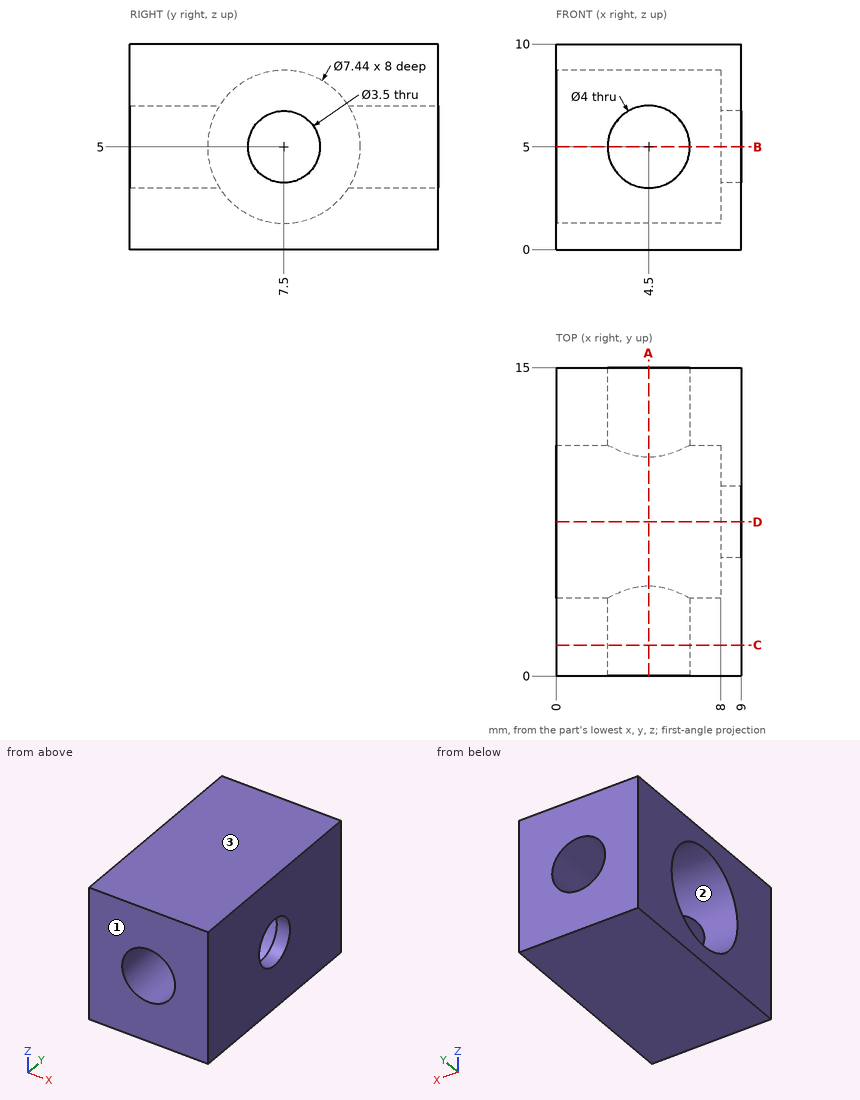
Print and shaded views of the part. All mm, measured from the part's lowest x, y and z. Coordinates: 2 decimals unless noted, no trailing zeros. Order: outer loops, then holes, each group sorted by start corner. A loop starts at its lowest first (then second) coordinate and runs counter-clockwise, first axis right, second up. Notation, with made-up numbers: (-21.5, 24.5) - (15.5, 24.5) arc R16 ccw to (15.5, 32.5) - close; hole circle Ø6 at (68.25, 5). An arc over 180 degrees is marked (long way). Return JSON: item names as keys, results as strings. Group by question number.
Item 1: Cut at C-C (y = 1.5). List the corners of the cut face in (x, z), plus the area to 3 significant figures.
Item 2: Cut at B-B (z = 5). List the corners of the cut face in (x, y), plus the area to 3 significant figures.
Item 3: Pull direction Y, two halves, no side cores. Call the marked faces 1, 2 and 3: pulls with the +Y half, pulls with the -Y half, needs draft (parallel to the pull), parting line crosses it, or undercut.
Item 4: Cut at A-A (x = 4.5). List the corners of the cut face in (y, z).
Item 5: Cut at D-D (y = 7.5). List the corners of the cut face in (x, z).
Item 6: Drill centre lines: probe 1 along X at (y, z) = (2.05, 5); probe 2 along Z at (x, y) = (4.5, 2.7); probe 3 along Z at (x, y) = (4.25, 7.5). Where is each one in solid material? Low to high. Write a range as from..to.
Item 7: Pin check, flat tips, straight feed: pin 1 (3.5 mm diameter, centred on x = 4.5, z = 5, fed in from -Y); pin 2 (4.5 mm diameter, centred on y = 7.5, z = 5, fed in from -X); pin 3 (4 mm diameter, centred on x = 2, y = 4, fed in from -Z). Stop position of each tip, or through.
Check values:
{
 "1": {"outline": "(0, 0) - (9, 0) - (9, 10) - (0, 10) - close; hole circle Ø4 at (4.5, 5)", "area": "77.4 mm2"},
 "2": {"outline": "(0, 0) - (2.5, 0) - (2.5, 3.78) - (0, 3.78) - close; (0, 11.22) - (2.5, 11.22) - (2.5, 15) - (0, 15) - close; (6.5, 0) - (9, 0) - (9, 5.75) - (8, 5.75) - (8, 3.78) - (6.5, 3.78) - close; (6.5, 11.22) - (8, 11.22) - (8, 9.25) - (9, 9.25) - (9, 15) - (6.5, 15) - close", "area": "41.7 mm2"},
 "3": {"face 1": "pulls with the -Y half", "face 2": "undercut", "face 3": "needs draft"},
 "4": {"outline": "(0, 0) - (15, 0) - (15, 3) - (10.64, 3) arc R3.72 cw to (4.36, 3) - (0, 3) - close; (0, 7) - (4.36, 7) arc R3.72 cw to (10.64, 7) - (15, 7) - (15, 10) - (0, 10) - close"},
 "5": {"outline": "(0, 0) - (9, 0) - (9, 3.25) - (8, 3.25) - (8, 1.28) - (0, 1.28) - close; (0, 8.72) - (8, 8.72) - (8, 6.75) - (9, 6.75) - (9, 10) - (0, 10) - close"},
 "6": {"probe 1": "x = 0..2.5, 6.5..9", "probe 2": "z = 0..3, 7..10", "probe 3": "z = 0..1.28, 8.72..10"},
 "7": {"pin 1": "passes through", "pin 2": "stops at x = 8", "pin 3": "stops at z = 0"}
}
